Answer from the drawing. Dimensions are ordinates in mm from the lowest x, y and z of the part. A direction names the side the tool comes from. Coordinates: 2 decimals unless noted, no trailing zeros. Write each loop counter-clockwise with the first axis right and the second up, starting at its lowest first coordinate (ties: lowest second). Pieces come first, ordered by that corner, then holes.
(1) Which of the six approach directions +Z, -Z, +X, -X, +Y, -Y give full straight-line access (tool end or side, diameter ignored) to the marked faces 1, 2, 3 and 4?
(2) Straight lines are drawn through the part: line 1 (Z direction, x = 38, y = 33); line 2 (X direction, y = 19.5, z = 61.5); line 3 (Z direction, x = 18.5, y = 40). For each, find the intervals that lie inside material, in ascending order.
(3) The part is cut by section A-A on x = 21.5. Determine the outline of the cut face in (y, z).
(4) Given P1, Ø6, axis at x = 27.5, y = 13.5, coming from the -Z side; P2, Ø5, axis at x = 11.5, y = 37.5, coming from the +Z side; P3, Ø2, axis at x = 22, z = 49.5, coming from the +Y side, each flat-ended and moving along its own axis, determine where each tip first touches the part or whether it passes through.
(5) The part is cut by section C-C on x = 43.5. Determine the outline of the cut face in (y, z).
(6) For a pull along X with two mould halves and no side action, classify the marked faces 5, 6 and 7 as +X half, -X half, draft (parallel to the pull), parting line (faces both ways), or undercut.
(7) The part is cut by section D-D on y = 24. Determine the outline of the cut face in (x, z).
(8) The part is cut by section B-B on y = 8. Determine the outline of the cut face in (x, z).
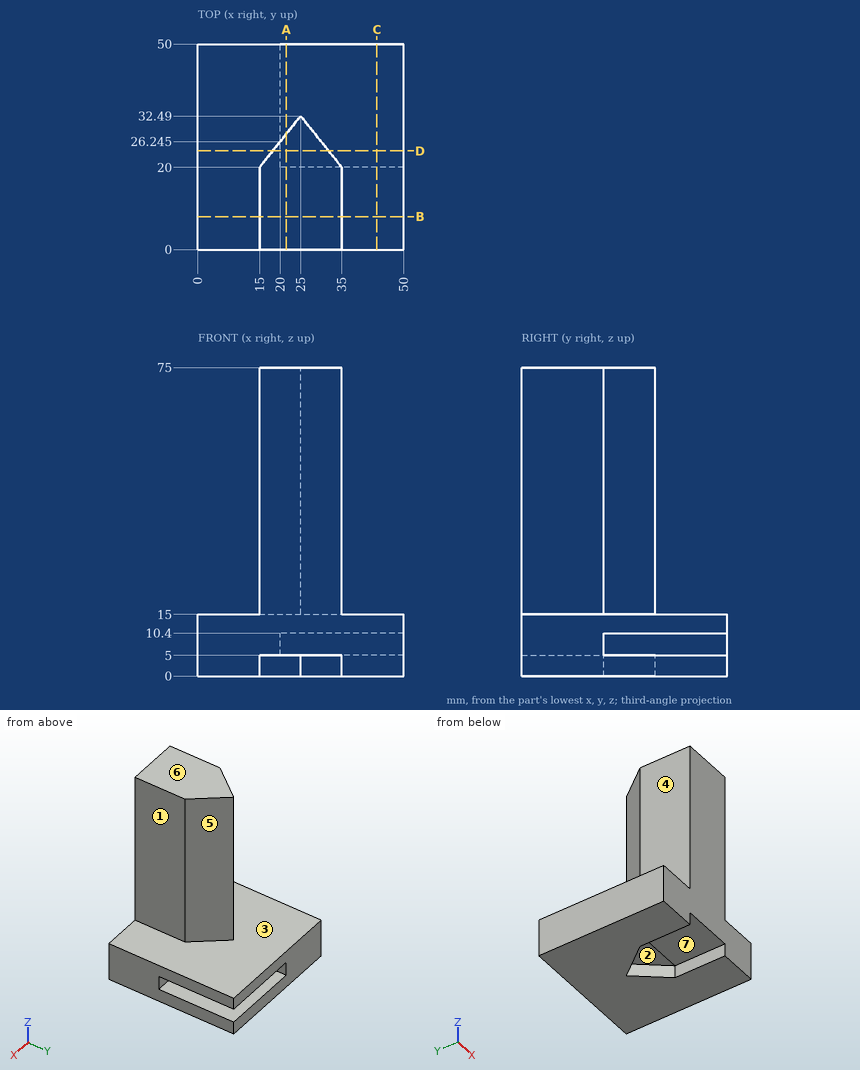
Model answer:
1. face 1: +Z, +X, +Y, -Y
1. face 2: +X, +Y
1. face 3: +Z, +Y
1. face 4: +Z, -X, +Y, -Y
2. line 1: z = 0 to 5, 10.4 to 15
2. line 2: x = 15 to 35
2. line 3: z = 0 to 15
3. outline: (0, 5) - (20, 5) - (20, 10.4) - (50, 10.4) - (50, 15) - (28.12, 15) - (28.12, 75) - (0, 75) - close; (28.12, 0) - (50, 0) - (50, 5) - (28.12, 5) - close
4. P1: stops at z = 5
4. P2: stops at z = 15
4. P3: stops at y = 29.99
5. outline: (0, 0) - (50, 0) - (50, 5) - (20, 5) - (20, 10.4) - (50, 10.4) - (50, 15) - (0, 15) - close
6. face 5: +X half
6. face 6: draft
6. face 7: undercut
7. outline: (0, 0) - (18.2, 0) - (18.2, 5) - (20, 5) - (20, 10.4) - (50, 10.4) - (50, 15) - (31.8, 15) - (31.8, 75) - (18.2, 75) - (18.2, 15) - (0, 15) - close; (31.8, 0) - (50, 0) - (50, 5) - (31.8, 5) - close
8. outline: (0, 0) - (15, 0) - (15, 5) - (35, 5) - (35, 0) - (50, 0) - (50, 15) - (35, 15) - (35, 75) - (15, 75) - (15, 15) - (0, 15) - close
